Read the model definition and answer for the solid it produces. Units are mm, in the model's axes. Face numbers are marked on the shaded views. A direction names the side the tool comes from. Round coordinates to 2 decimals unless told otherwise and drop trailing zeros. Order: outer loops, then holes, each group sorted by start corner. A loop starts at its lowest first (then second) coordinate and runs counter-clockwise, first axis right, second up. Notation, with made-up numbers: (52, -10) -> (101, -10) arc R31 ccw to (101, 20) -> close; hole circle Ø6 at (15.5, -8). An arc over 180 degrees is marked (long way). Use a Markdown table: item, result. Add a question column.
1. Consider L1, parallel to X at y = 74, z = 23; L2, parallel to Y at x = 126, z = 7 (3 decimals); L3, parallel to X at y = 32, z = 9. Determine where each line is inside the solid, lowest interval first. Write a range as [from, to].
2. The mould has two halves that part along Z. Classify the marked faces 4, 5 and 6: +Z half, -Z half, draft (parallel to the pull), parting line (faces both ways), or undercut.
3. Section C-C, the plane y = 9 is taken. Give the vertices of the cut face in (x, z).
4. Section A-A, the plane z = 15 is taken. Give the vertices of the cut face in (x, y) (3 decimals).
5. For the marked faces 1, 2 and 3, determine the directions among +Z, -Z, +X, -X, +Y, -Y from which every point of the face is accessible in a straight line to the end or side of a thin tool.
6. Section B-B, the plane x = 25.5 is taken. Give the vertices of the cut face in (y, z) (3 decimals), then the cut area to 3 significant figures.
7. Given pin 1 (3 mm diameter, centred on x = 28, z = 8, fed in from -Y); pin 2 (8 mm diameter, centred on x = 145.5, y = 107.5, fed in from +Z); pin 3 (8 mm diameter, centred on x = 53, y = 36.5, fed in from -Z); pin 4 (3.5 mm diameter, centred on x = 149, y = -5.5, fed in from +Z), each flat-ended and moving along its own axis, determine where each tip first touches the part or whether it passes through.
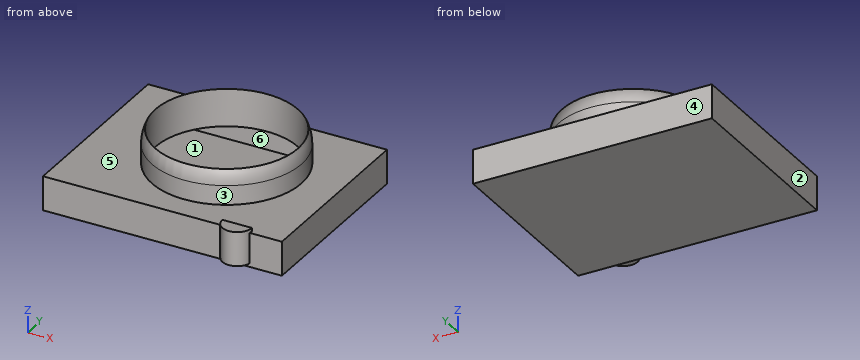
```python
from build123d import *

# Parameters (mm, degrees)
F0_W     = 178.1788319349
F0_H     = 140.1249915361
F1_DEPTH = 25.4
F2_R     = 55.7882871659
F3_DEPTH = 25.4
F4_T     = -2.54
F7_DEPTH = 25.4


# Not quite as in the source:
# - a fillet or chamfer that OpenCascade refuses, or shapes differently, is made with other operations: its cross-section is extruded or revolved along the edge and cut away or added


with BuildPart() as f1:
    # F0 (on Top) → F1 (new body)
    with BuildSketch(Plane.XY):
        with Locations((89.0894159675, 70.0624957681)):
            Rectangle(F0_W, F0_H)
    extrude(amount=F1_DEPTH)

    # F2 (on face) → F3 (join)
    with BuildSketch(Plane.XY.offset(25.4)):
        with Locations((95.6915691495, 73.8431587815)):
            Circle(F2_R)
    extrude(amount=F3_DEPTH)

    # F4
    f4_openings = [f1.faces().sort_by_distance(p)[0] for p in [
        (95.691569, 73.843159, 50.8),
    ]]
    offset(amount=F4_T, openings=f4_openings, kind=Kind.INTERSECTION)

    # F5: fillet of radius 25.4 on 1 edges, made by hand

    # F5_s1 → F5_t2 (revolve, cut)
    with BuildSketch(Plane.XZ.offset(-73.8431587815)):
        with BuildLine():
            ThreePointArc((151.4798563154, 39.7283966834), (150.8367139512, 45.4080093463), (148.9398563154, 50.8))
            Line((148.9398563154, 50.8), (151.4798563154, 50.8))
            Line((151.4798563154, 50.8), (151.4798563154, 39.7283966834))
        make_face()
    revolve(axis=Axis((95.6915691495, 73.8431587815, 50.8), (0, 0, 1)), mode=Mode.SUBTRACT)

    # F6 (on face) → F7 (join)
    with BuildSketch(Plane.XY.offset(2.54)):
        with BuildLine():
            ThreePointArc((132.352274685, 2.54), (143.3852910995, -8.4930164146), (154.4183075141, 2.54))
            Line((154.4183075141, 2.54), (132.352274685, 2.54))
        make_face()
    extrude(amount=F7_DEPTH)


solid = f1.part
```
Verdict:
| question | item | result |
|---|---|---|
| 1 | L1 | x = [0, 42.44], [148.94, 178.18] |
| 1 | L2 | y = [0, 2.54], [137.585, 140.125] |
| 1 | L3 | x = [0, 2.54], [175.64, 178.18] |
| 2 | face 4 | draft |
| 2 | face 5 | +Z half |
| 2 | face 6 | undercut |
| 3 | outline | (0, 0) -> (178.18, 0) -> (178.18, 25.4) -> (0, 25.4) -> close; hole (2.54, 2.54) -> (175.64, 2.54) -> (175.64, 22.86) -> (2.54, 22.86) -> close |
| 4 | outline | (0, 0) -> (132.649, 0) arc R11.033 ccw to (154.122, 0) -> (178.179, 0) -> (178.179, 140.125) -> (0, 140.125) -> close; hole (2.54, 2.54) -> (175.639, 2.54) -> (175.639, 137.585) -> (2.54, 137.585) -> close |
| 5 | face 1 | none |
| 5 | face 2 | +Z, -Z, -X, +Y, -Y |
| 5 | face 3 | +Z |
| 6 | outline | (0, 0) -> (140.125, 0) -> (140.125, 25.4) -> (0, 25.4) -> close; hole (2.54, 2.54) -> (137.585, 2.54) -> (137.585, 22.86) -> (2.54, 22.86) -> close |
| 6 | area | 815 mm2 |
| 7 | pin 1 | stops at y = 0 |
| 7 | pin 2 | stops at z = 25.4 |
| 7 | pin 3 | stops at z = 0 |
| 7 | pin 4 | stops at z = 27.94 |
